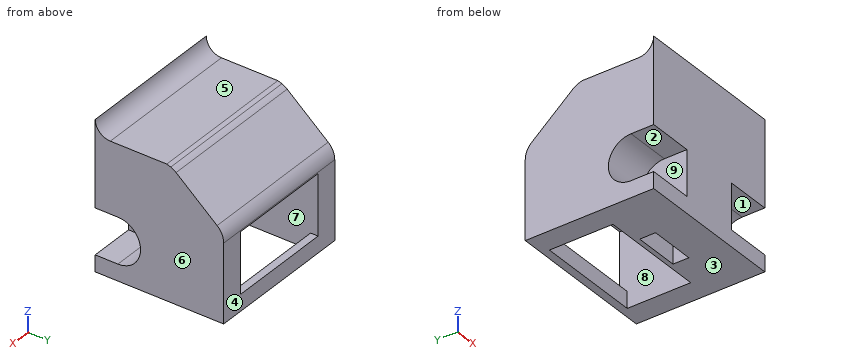
Autodesk Inventor part; units mm, degrees
ref_plane "YZ Plane" through (0, 0, 0) normal (1, 0, 0) x (0, 1, 0)
ref_plane "XZ Plane" through (0, 0, 0) normal (0, 1, 0) x (-1, 0, 0)
ref_plane "XY Plane" through (0, 0, 0) normal (0, 0, 1) x (1, 0, 0)
sketch "Esboço1" plane through (0, 0, 0) normal (0, 1, 0) x (-1, 0, 0)
  line L0 (0, 0) -> (-100, 0)
  line L1 (-100, 0) -> (-100, -100)
  line L2 (-100, -100) -> (0, -100)
  line L3 (0, -100) -> (0, 0)
  dimension "d0" = 100
  dimension "d1" = 100
extrude "Extrusão1" add sketch "Esboço1" along normal blind 85
sketch "Esboço2" plane through (100, 0, 0) normal (1, 0, 0) x (0, 0, -1)
  line L0 (0, 0) -> (100, 0)
  line L1 (0, 0) -> (2.5, 0)
  line L2 (12.5, 10) -> (12.5, 45.3759)
  line L3 (0, 85) -> (100, 85)
  line L4 (12.5, 50) -> (13.3867, 50)
  line L5 (42.5, 85) -> (12.5, 85)
  line L6 (12.5, 85) -> (12.5, 50)
  line L7 (15.5093, 53.5108) -> (38.7585, 80.6349)
  arc A0 (2.5, 0) -> (12.5, 10) centre (2.5, 10) ccw
  line L8 (2.5, 0) -> (100, 0)
  line L9 (48.2492, 85) -> (100, 85)
  line L10 (100, 85) -> (100, 0)
  arc A1 (15.5093, 53.5108) -> (12.5, 45.3759) centre (25, 45.3759) ccw
  line L11 (12.5, 85) -> (42.5, 85)
  line L12 (12.5, 85) -> (0, 85)
  arc A2 (48.2492, 85) -> (38.7585, 80.6349) centre (48.2492, 72.5) ccw
  circle A3 centre (74.1246, 15) radius 15
  line L13 (0, 85) -> (0, 0)
  line L14 (0, 0) -> (2.5, 0)
  line L15 (59.1246, 15) -> (59.1246, 0)
  line L16 (89.1246, 15) -> (89.1246, 0)
  line L17 (12.5, 50) -> (12.5, 45.3759)
  line L18 (12.5, 85) -> (48.2492, 85)
  point P0 (12.5, 0)
  dimension "d4" = 12.5
  dimension "d7" = 10
  dimension "d8" = 12.5
  dimension "d9" = 12.5
  dimension "d11" = 30
extrude "Extrusão2" cut sketch "Esboço2" against normal blind 100 contours L13 L3 L6 L17 L2 A0 L0 | L3 A2 L7 A1 L4 L6
extrude "Extrusão3" cut sketch "Esboço2" against normal blind 30 contours L15 A3 L0 | A3 L16 L0 | A3
sketch "Esboço3" plane through (0, 0, -100) normal (-1, 0, 0) x (0, 0, 1)
  line L0 (86.6133, 50) -> (87.5, 50)
  arc A0 (86.6133, 50) -> (84.4907, 53.5108) centre (75, 45.3759) ccw
  line L1 (86.6133, 50) -> (87.5, 47.3246)
  line L2 (87.5, 50) -> (87.5, 10)
  line L3 (86.6133, 50) -> (87.5, 50)
  line L4 (87.5, 50) -> (87.5, 47.3246)
  arc A1 (40.8754, 15) -> (10.8754, 15) centre (25.8754, 15) ccw
  circle A2 centre (25.8754, 15) radius 15
  line L5 (10.8754, 15) -> (10.8754, 0)
  line L6 (10.8754, 15) -> (10.8754, 0)
  line L7 (97.5, 0) -> (40.8754, 0)
  line L8 (40.8754, 15) -> (40.8754, 0)
  line L9 (10.8754, 0) -> (40.8754, 0)
  point P0 (100, 0)
extrude "Extrusão4" cut sketch "Esboço3" against normal blind 30 contours A2 A1 | L8 L9 A2 | A2 L9 L5
extrude "Extrusão5" cut sketch "Esboço3" against normal blind 100 contours L0 L2 L1
sketch "Esboço4" plane through (100, 0, -100) normal (0, 0, -1) x (-1, 0, 0)
  line L0 (15, 35) -> (85, 35)
  line L1 (15, 35) -> (15, 80)
  line L2 (0, 53.5108) -> (100, 53.5108)
  line L3 (15, 35) -> (60, 35) construction
  line L4 (15, 80) -> (85, 80)
  line L5 (85, 80) -> (85, 35)
  line L6 (70, 30) -> (70, 15)
  line L7 (15, 35) -> (15, 38)
  line L8 (15, 38) -> (85, 38)
  line L9 (0, 0) -> (0, 85)
  line L10 (0, 35) -> (50, 35)
  line L11 (37.5, 35) -> (35, 35)
  line L12 (35, 35) -> (35, 22.5)
  line L13 (35, 22.5) -> (65, 22.5)
  line L14 (65, 22.5) -> (65, 35)
  line L15 (35, 22.5) -> (35, 24.5)
  line L16 (35, 24.5) -> (65, 24.5)
  dimension "d26" = 70
  dimension "d27" = 45
  dimension "d31" = 3
  dimension "d34" = 30
  dimension "d35" = 2
extrude "Extrusão6" cut sketch "Esboço4" against normal blind 60 contours L0 L14 L16 L12 | L1 L2 L5 L8 | L1 L4 L5 L2
sketch "Esboço5" plane through (0, 85, 0) normal (0, 1, 0) x (1, 0, 0)
  line L0 (100, 89.1246) -> (70, 89.1246)
  line L1 (85, 89.1246) -> (85, 49.1246)
  line L2 (85, 100) -> (85, 40)
  line L3 (85, 49.1246) -> (15, 49.1246)
  line L4 (15, 100) -> (15, 40)
  line L5 (15, 49.1246) -> (15, 89.1246)
  line L6 (15, 89.1246) -> (85, 89.1246)
  point P0 (0, 0)
  dimension "d38" = 40
extrude "Extrusão7" cut sketch "Esboço5" against normal blind 30
properties part number "Mini-sumô rascunho"
Here's how the part is built. I have some questions about the finished solid (model axes, mm). Face numbers are marked on the shaded views. A direction names the side the tool comes from. Round coordinates to 2 decimals unless told otherwise and drop trailing zeros. Write each loop counter-clockwise with the first axis right and the second up, starting at its lowest first coordinate (ties: lowest second). Pieces come first, ordered by that corner, then holes.
1. I need wall thicknesses on L1, parallel to Y at x = 52.5, z = -91; L2, parallel to X at y = 27, z = -66.5; L3, parallel to X at y = 68, z = -65. Which ranges of each line are inside material? Lowest first, please.
2. For the marked faces 1, 2, 3, 4 and 5, which set-ups out of +Z, -Z, +X, -X, +Y, -Y let a thin tool reach every point of the face, with its end or its side?
3. Suppose I cut it at A-A (x = 56). List the corners of the cut face in (y, z) for me.
4. If we mould it in two halves opening along X, with no side actions, what happens to the marked faces 6, 7, 8 and 9? For each: released by +X, released by -X, zero draft, split by the parting line, or undercut.
5. Will these pins go through, and if not, where does the flat tip stop? pin 1 Ø18 at (x, z) = (55.5, -78) entering from +Y; pin 2 Ø2 at (x, y) = (68.5, 49.5) entering from +Z; pin 3 Ø21 at (x, y) = (46.5, 53) entering from -Z; pin 4 Ø1 at (y, z) = (76, -31.5) entering from +X.
6. Suppose I cut it at B-B (z = -77). List the corners of the cut face in (x, y) for me, and give its area (3 significant figures).
7. Suppose I cut it at D-D (y = 52). List the corners of the cut face in (x, z) for me, and give its area (3 significant figures).
8. Suppose I cut it at C-C (x = 12.5). List the corners of the cut face in (y, z) for me, and give its area (3 significant figures).
Answer sheet:
1. L1: y = 0 to 24.5, 35 to 38, 80 to 85
1. L2: x = 30 to 35, 65 to 70
1. L3: x = 0 to 15, 85 to 100
2. face 1: +X, -Y
2. face 2: -X, -Y
2. face 3: -Z, +X, -X, +Y, -Y
2. face 4: +Z, -Z, +X, -X, +Y
2. face 5: +Z, +X, -X, +Y
3. outline: (0, -100) - (24.5, -100) - (24.5, -40) - (35, -40) - (35, -100) - (38, -100) - (38, -40) - (80, -40) - (80, -49.12) - (85, -49.12) - (85, -48.25) arc R12.5 ccw to (80.63, -38.76) - (53.51, -15.51) arc R12.5 ccw to (50, -13.39) - (47.32, -12.5) - (10, -12.5) arc R10 cw to (0, -2.5) - close; (80, -100) - (85, -100) - (85, -89.12) - (80, -89.12) - close
4. face 6: released by +X
4. face 7: undercut
4. face 8: undercut
4. face 9: released by -X
5. pin 1: stops at y = 38
5. pin 2: stops at z = -12.89
5. pin 3: stops at z = -40
5. pin 4: passes through
6. outline: (0, 29.72) - (30, 29.72) - (30, 0) - (70, 0) - (70, 29.72) - (100, 29.72) - (100, 85) - (85, 85) - (85, 38) - (15, 38) - (15, 85) - (0, 85) - close; hole (35, 24.5) - (65, 24.5) - (65, 35) - (35, 35) - close
6. area: 3,110 mm2
7. outline: (0, -100) - (15, -100) - (15, -40) - (85, -40) - (85, -100) - (100, -100) - (100, -14.4) - (0, -14.4) - close
7. area: 4,360 mm2
8. outline: (0, -100) - (85, -100) - (85, -48.25) arc R12.5 ccw to (80.63, -38.76) - (53.51, -15.51) arc R12.5 ccw to (50, -13.39) - (47.32, -12.5) - (10, -12.5) arc R10 cw to (0, -2.5) - (0, -59.12) - (15, -59.12) arc R15 cw to (15, -89.12) - (0, -89.12) - close
8. area: 6,120 mm2
